Here's the drawing with two shaded views (mm, measured from the low corner). I have some questions. Round coordinates to 2 decimals unless told otherwise and drop trailing zeros. Write each loop counter-clockwise with the first axis right and the second up, starting at its lowest first coordinate (ties: lowest second). Pieces come first, ordered by that corner, then holes. Notation, with made-up numbers: (-18, 74) -> (2, 74) arc R15 cw to (2, 96) -> close; hole circle Ø11 at (-14.5, 69). An arc over 180 degrees is marked (long way). Use CSV: the item, a comma, the result in double quotes.
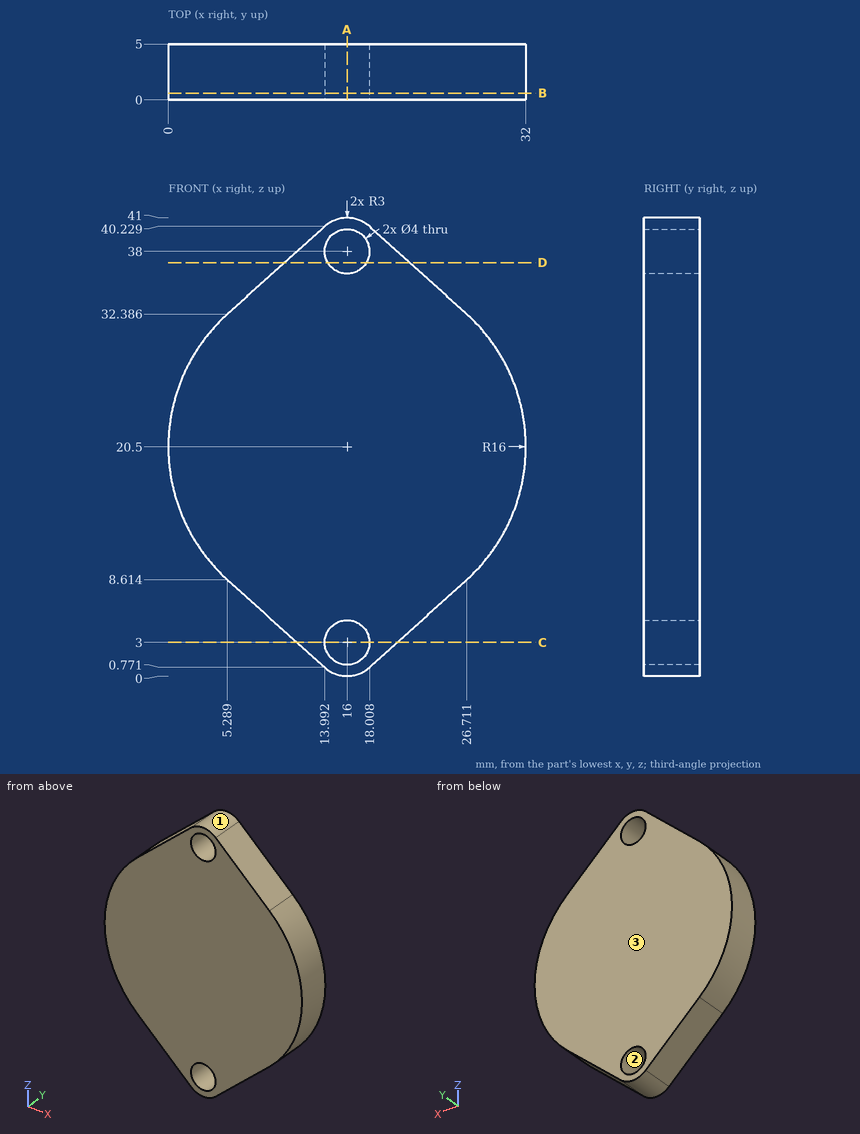
Q1. Suppose I cut it at C-C (z = 3). Write out the boundary of the cut face in (x, y).
Resolved:
outline,"(11.52, 0) -> (14, 0) -> (14, 5) -> (11.52, 5) -> close; (18, 0) -> (20.48, 0) -> (20.48, 5) -> (18, 5) -> close"
Q2. Suppose I cut it at A-A (x = 16). Write out the boundary of the cut face in (y, z), and give its area (3 significant figures).
Resolved:
outline,"(0, 0) -> (5, 0) -> (5, 1) -> (0, 1) -> close; (0, 5) -> (5, 5) -> (5, 36) -> (0, 36) -> close; (0, 40) -> (5, 40) -> (5, 41) -> (0, 41) -> close"
area,"165 mm^2"
Q3. Suppose I cut it at B-B (y = 0.6). Write out the boundary of the cut face in (x, z) (1 decimal), and give its area (3 significant figures).
Resolved:
outline,"(5.3, 8.6) -> (14, 0.8) arc R3 ccw to (18, 0.8) -> (26.7, 8.6) arc R16 ccw to (26.7, 32.4) -> (18, 40.2) arc R3 ccw to (14, 40.2) -> (5.3, 32.4) arc R16 ccw to start; hole circle Ø4 at (16, 3); hole circle Ø4 at (16, 38)"
area,"862 mm^2"
Q4. Will these pins go through, and if not, where does the flat tip stop? P1, Ø3, axis at x = 9, y = 1, coming from the +Z side; P2, Ø1, axis at y = 0.5, z = 23, coming from the +X side (1 decimal); P3, Ø2, axis at y = 1, z = 31, coming from the +X side (1 decimal).
Resolved:
P1,"stops at z = 37.08"
P2,"stops at x = 31.9"
P3,"stops at x = 28.9"
Q5. Suppose I cut it at D-D (z = 37). Write out the boundary of the cut face in (x, y), and give its area (3 significant figures).
Resolved:
outline,"(10.41, 0) -> (14.27, 0) -> (14.27, 5) -> (10.41, 5) -> close; (17.73, 0) -> (21.59, 0) -> (21.59, 5) -> (17.73, 5) -> close"
area,"38.6 mm^2"
Q6. If we mould it in two halves opening along X, with no side actions, what happens to the marked faces 1, 2 and 3? For each: released by +X, released by -X, zero draft, split by the parting line, or undercut.
Resolved:
face 1,"split by the parting line"
face 2,"undercut"
face 3,"zero draft"
Q7. Please list where these lines run through material, in increasing order: probe 1 along X at (y, z) = (2.55, 3); probe 2 along Z at (x, y) = (11, 2.65); probe 3 along Z at (x, y) = (24, 2.6).
Resolved:
probe 1,"x = 11.52 to 14, 18 to 20.48"
probe 2,"z = 3.47 to 37.53"
probe 3,"z = 6.17 to 34.83"
